Can you work these out from the drawing? Everything is in mm from the part's minimum corner. Coordinates: 2 decimals unless noted, no trailing zeros. Loops run counter-clockwise (first coordinate to the right, second up) from the corner with the lowest first, then second, coordinate; pieces in that order, holes last. Notation, with made-up numbers: (51, -38) -> (102, -38) arc R29 ccw to (102, -8) -> close; hole circle Ø4 at (57.25, 88). An arc over 180 degrees is marked (long way). One line per question, with ' | ' between items.
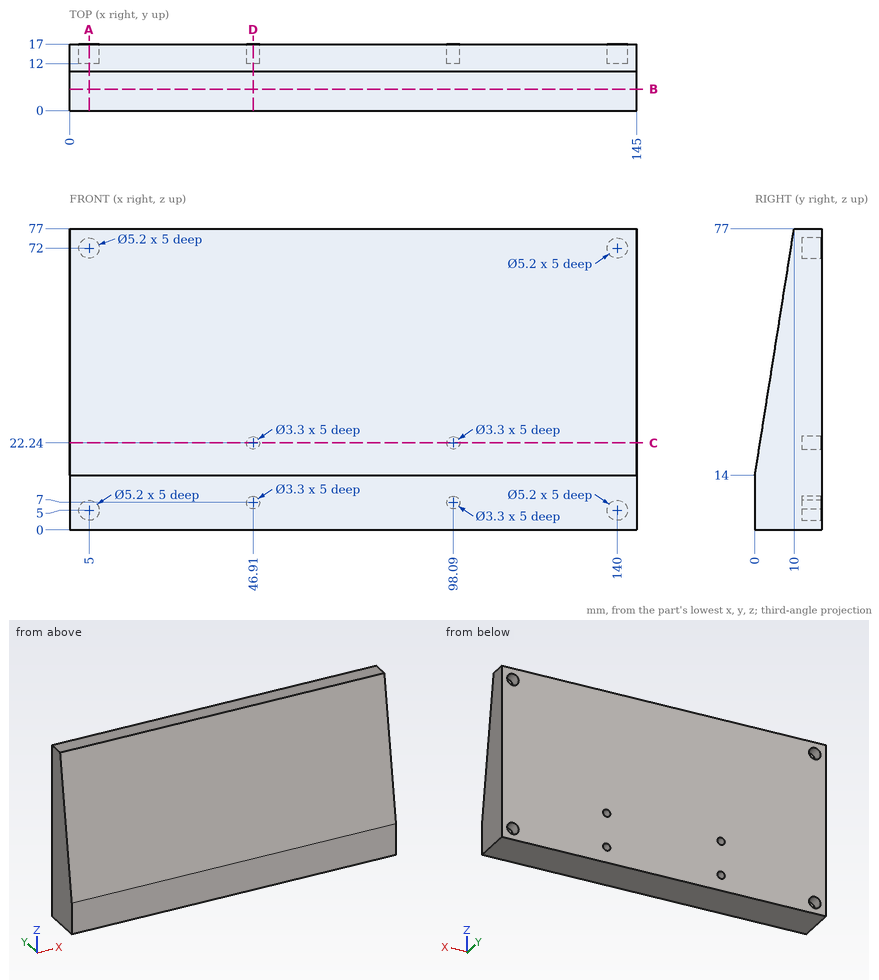
Q1. For pin 1 (1 mm diameter, centred on x = 98, z = 22.5, fed in from +Y), with a flat end and sliding along its axis, tell me the tip position at first contact or that it passes through.
Values follow:
pin 1: stops at y = 12
Q2. Imagine slicing it at D-D on x = 46.91. Write out the boundary of the cut face in (y, z), plus the area to 3 significant figures.
Values follow:
outline: (0, 0) -> (17, 0) -> (17, 5.35) -> (12, 5.35) -> (12, 8.65) -> (17, 8.65) -> (17, 20.59) -> (12, 20.59) -> (12, 23.89) -> (17, 23.89) -> (17, 77) -> (10, 77) -> (0, 14) -> close | area: 961 mm2
Q3. Please list where these lines run through material, in increasing order: L1, parallel to X at y = 13.1, z = 22.24; L2, parallel to X at y = 15.35, z = 5; L3, parallel to Z at x = 46.91, y = 13.65. Write a range as [from, to].
Values follow:
L1: x = [0, 45.26], [48.56, 96.44], [99.74, 145] | L2: x = [0, 2.4], [7.6, 137.4], [142.6, 145] | L3: z = [0, 5.35], [8.65, 20.59], [23.89, 77]
Q4. Imagine slicing it at C-C on z = 22.24. Write out the boundary of the cut face in (x, y).
Values follow:
outline: (0, 1.31) -> (145, 1.31) -> (145, 17) -> (99.74, 17) -> (99.74, 12) -> (96.44, 12) -> (96.44, 17) -> (48.56, 17) -> (48.56, 12) -> (45.26, 12) -> (45.26, 17) -> (0, 17) -> close
Q5. Imagine slicing it at A-A on x = 5. Write out the boundary of the cut face in (y, z), plus the area to 3 significant figures.
Values follow:
outline: (0, 0) -> (17, 0) -> (17, 2.4) -> (12, 2.4) -> (12, 7.6) -> (17, 7.6) -> (17, 69.4) -> (12, 69.4) -> (12, 74.6) -> (17, 74.6) -> (17, 77) -> (10, 77) -> (0, 14) -> close | area: 942 mm2
Q6. Imagine slicing it at B-B on y = 5.5. Write out the boundary of the cut face in (x, z).
Values follow:
outline: (0, 0) -> (145, 0) -> (145, 48.65) -> (0, 48.65) -> close
